```python
from build123d import *

# Parameters (mm, degrees)
F0_R     = 1.4605
F1_DEPTH = 6.35


# Not quite as in the source:
# - a feature names something its author has since deleted; it is built from what else it names


with BuildPart() as f1:
    # F0 (on Top) → F1 (new body)
    with BuildSketch(Plane.XY):
        Polygon((-57.1500000004, 101.5999999999), (-76.2, 101.5999999999), (-76.2, 40.4022223395), (-73.2282, 40.4022223395), (-73.2282, 32.3377223395), (-65.6082, 32.3377223395), (-65.6082, 34.0522223395), (-63.1952, 34.0522223395), (-63.1952, 32.3377223395), (-55.5752, 32.3377223395), (-55.5752, 30.8772223395), (-55.5752, 29.4167223395), (-63.1952, 29.4167223395), (-63.1952, 27.7022223395), (-65.6082, 27.7022223395), (-65.6082, 29.4167223395), (-73.2282, 29.4167223395), (-73.2282, 21.3522223395), (-76.2, 21.3522223395), (-76.2, -16.7477776605), (-73.2282, -16.7477776605), (-73.2282, -24.8122776605), (-65.6082, -24.8122776605), (-65.6082, -23.0977776605), (-63.1952, -23.0977776605), (-63.1952, -24.8122776605), (-55.5752, -24.8122776605), (-55.5752, -26.2727776605), (-55.5752, -27.7332776605), (-63.1952, -27.7332776605), (-63.1952, -29.4477776605), (-65.6082, -29.4477776605), (-65.6082, -27.7332776605), (-73.2282, -27.7332776605), (-73.2282, -35.7977776604), (-76.2, -35.7977776604), (-76.2, -101.5999999999), (76.2, -101.5999999999), (76.2, -35.7977776604), (73.2282, -35.7977776604), (73.2282, -27.7332776605), (65.6082, -27.7332776605), (65.6082, -29.4477776605), (63.1952, -29.4477776605), (63.1952, -27.7332776605), (55.5752, -27.7332776605), (55.5752, -26.2727776605), (55.5752, -24.8122776605), (63.1952, -24.8122776605), (63.1952, -23.0977776605), (65.6082, -23.0977776605), (65.6082, -24.8122776605), (73.2282, -24.8122776605), (73.2282, -16.7477776605), (76.2, -16.7477776605), (76.2, 21.3522223395), (73.2282, 21.3522223395), (73.2282, 29.4167223395), (65.6082, 29.4167223395), (65.6082, 27.7022223395), (63.1952, 27.7022223395), (63.1952, 29.4167223395), (55.5752, 29.4167223395), (55.5752, 30.8772223395), (55.5752, 32.3377223395), (63.1952, 32.3377223395), (63.1952, 34.0522223395), (65.6082, 34.0522223395), (65.6082, 32.3377223395), (73.2282, 32.3377223395), (73.2282, 40.4022223395), (76.2, 40.4022223395), (76.2, 101.5999999999), (57.1499999998, 101.5999999999), (57.1499999998, 98.6281999999), (39.5605000002, 98.6281999999), (39.5605000002, 91.0081999999), (41.2750000002, 91.0081999999), (41.2750000002, 88.5951999999), (39.5605000002, 88.5951999999), (39.5605000002, 80.9751999999), (38.1000000002, 80.9751999999), (36.6395000002, 80.9751999999), (36.6395000002, 88.5951999999), (34.9250000002, 88.5951999999), (34.9250000002, 91.0081999999), (36.6395000002, 91.0081999999), (36.6395000002, 98.6281999999), (19.05, 98.6281999999), (19.05, 101.5999999999), (-19.05, 101.5999999999), (-19.05, 98.6281999999), (-21.3974503974, 98.6281999999), (-36.6395000002, 98.6281999999), (-36.6395000002, 91.0081999999), (-34.9250000002, 91.0081999999), (-34.9250000002, 88.5951999999), (-36.6395000002, 88.5951999999), (-36.6395000002, 80.9751999999), (-38.1000000002, 80.9751999999), (-39.5605000002, 80.9751999999), (-39.5605000002, 88.5951999999), (-41.2750000002, 88.5951999999), (-41.2750000002, 91.0081999999), (-39.5605000002, 91.0081999999), (-39.5605000002, 98.6281999999), (-57.1500000004, 98.6281999999), align=None)
        with BuildLine():
            add(Edge.make_bspline(
                [(12.7658935974, -21.8633876268), (13.9035680881, -23.0010621174), (13.9035680881, -25.0432889762)],
                knots=[0, 0, 0, 1, 1, 1], degree=2))
            add(Edge.make_bspline(
                [(13.9035680881, -25.0432889762), (13.9035680881, -27.2223065019), (12.7206178133, -28.3753940255)],
                knots=[0, 0, 0, 1, 1, 1], degree=2))
            add(Edge.make_bspline(
                [(12.7206178133, -28.3753940255), (11.5376675385, -29.5284815491), (9.3162641723, -29.5284815491)],
                knots=[0, 0, 0, 1, 1, 1], degree=2))
            Line((9.3162641723, -29.5284815491), (6.8771517165, -29.5284815491))
            Line((6.8771517165, -29.5284815491), (6.8771517165, -20.7257131361))
            Line((6.8771517165, -20.7257131361), (9.5744324733, -20.7257131361))
            add(Edge.make_bspline(
                [(9.5744324733, -20.7257131361), (11.6282191068, -20.7257131361), (12.7658935974, -21.8633876268)],
                knots=[0, 0, 0, 1, 1, 1], degree=2))
        make_face(mode=Mode.SUBTRACT)
        Polygon((21.2016391646, -28.6017729462), (21.2016391646, -29.5284815491), (15.1500971236, -29.5284815491), (15.1500971236, -28.7270038385), (19.8221727203, -21.6466418517), (15.294594307, -21.6466418517), (15.294594307, -20.7257131361), (21.0687017558, -20.7257131361), (21.0687017558, -21.5271908467), (16.3966261591, -28.6017729462), align=None, mode=Mode.SUBTRACT)
        with Locations((-74.5805352926, 2.3022223395)):
            Circle(F0_R, mode=Mode.SUBTRACT)
        with Locations((74.5805352926, 2.3022223395)):
            Circle(F0_R, mode=Mode.SUBTRACT)
        with Locations((0, 100.0089123845)):
            Circle(F0_R, mode=Mode.SUBTRACT)
    extrude(amount=F1_DEPTH)


solid = f1.part
```
Part model, mm, in its own coordinate system. A direction names the side the tool comes from. Round coordinates to 2 decimals unless told otherwise and drop trailing zeros.
Item 1: Drill centre lines: line 1 (Y direction, x = -57.5, z = 6); line 2 (Y direction, x = -57, z = 2.25); line 3 (X direction, y = 87, z = 4.5). Where is each one in solid material? Low to high.
Item 2: Drop flat-ended pins along their axis: P1, Ø0.9, axis at y = 28, z = 2.5, coming from the +X side; P2, Ø0.9, axis at x = -38, z = 2, coming from the +Y side; P3, Ø0.9, axis at y = -24, z = 4, coming from the -X side. Give the stop position or say it passes through.
Item 3: 3-axis set-ups, long thin cutter, end or side, ignore diameter. For faces 4 (the face through (59, 29.417, 3)), 5 (the face through (17.45, -25.24, 3.13)), 6 (the face through (-36.64, 85, 3)): which of +Z, -Z, +X, -X, +Y, -Y reach the whole face in a straight line?
Item 4: Cut at A-A, the plane z = 4.25. State how many separate pieces and enclosed holes the cut face has, then the cut area to 3 significant figures.
Item 5: Mould opens along Y. For faces 1 (the face through (-1, -101.6, 3)), 2 (the face through (39.561, 95, 3)), 3 (the face through (59, -24.812, 3)) say: +Y half, -Y half, draft (parallel to the pull), parting line (faces both ways), or undercut.
A:
1. line 1: y = -101.6 to -27.73, -24.81 to 29.42, 32.34 to 101.6
1. line 2: y = -101.6 to -27.73, -24.81 to 29.42, 32.34 to 98.63
1. line 3: x = -76.2 to -39.56, -36.64 to 36.64, 39.56 to 76.2
2. P1: stops at x = 73.23
2. P2: stops at y = 80.98
2. P3: stops at x = -73.23
3. face 4: +Z, -Z, +X
3. face 5: +Z, -Z
3. face 6: +Z, -Z, +Y
4. separate pieces: 1
4. enclosed holes: 5
4. area: 30,100 mm2
5. face 1: -Y half
5. face 2: draft
5. face 3: undercut
